Geometry: final body of the model. Coordinates: model frame, mm. Round coordinates to 2 decimals unless told otherwise and drop trailing zeros. Write each loop counter-clockwise with the first axis right and the second up, starting at its lowest first coordinate (ties: lowest second). Pieces come first, ordered by that corner, then holes. Notation, with made-up numbers: (45.25, -1) -> (96.25, -1) arc R12 ccw to (96.25, 12) -> close; hole circle Ø6 at (7.25, 74.25). An arc over 180 degrees is marked (long way). Use one line per item in the form item = value. Start each with the question number.
1. Cut plane B-B, the plane x = 1137.5. Return the cut outline in (y, z) (3 decimals), plus the area to 3 significant figures.
2. Pin query (flat end, axial travel): pin 1 Ø0.6 at (x, z) = (1142.5, 568) entering from +Y; pin 2 Ø3 at (x, y) = (1138, 34) entering from -Z; pin 3 Ø10 at (x, z) = (1132.5, 235.5) entering from -Y. Return the tip coordinate at first contact, or that it passes through.
3. Line query: L1, parallel to X at y = 27, z = 385.5; L2, parallel to Y at x = 1136.75, z = -371 (3 decimals); L3, parallel to Y at x = 1125.5, z = -221.5. Output: solid intervals per line, ascending.
```python
from build123d import *

# Parameters (mm, degrees)
EXTRUDE1_DEPTH     = 599.28125
CUT_EXTRUDE1_DEPTH = 25.4
CUT_EXTRUDE2_DEPTH = 25.4
CUT_EXTRUDE3_DEPTH = 25.4
SKETCH5_W          = 4.7625
SKETCH5_H          = 4.7625
CUT_EXTRUDE4_DEPTH = 0.79375
FILLET1_R          = 6.35


with BuildPart() as part:
    # Sketch1 → Extrude1 (new body, symmetric)
    with BuildSketch(Plane.XY):
        with BuildLine():
            Line((1143, 0), (1142.20625, 0))
            Line((1142.20625, 0), (1142.20625, 32.54375))
            ThreePointArc((1142.20625, 32.54375), (1141.741282015, 33.666282015), (1140.61875, 34.13125))
            Line((1140.61875, 34.13125), (1128.140506397, 34.13125))
            Line((1128.140506397, 34.13125), (1123.091401986, 31.071186722))
            Line((1123.091401986, 31.071186722), (1122.68, 31.75))
            Line((1122.68, 31.75), (1127.91875, 34.925))
            Line((1127.91875, 34.925), (1140.61875, 34.925))
            ThreePointArc((1140.61875, 34.925), (1142.302548023, 34.227548023), (1143, 32.54375))
            Line((1143, 32.54375), (1143, 0))
        make_face()
    extrude(amount=EXTRUDE1_DEPTH, both=True)

    # Sketch2 → Cut-Extrude1 (cut)
    with BuildSketch(Plane(origin=(1143, 0, 0), x_dir=(0, 0, -1), z_dir=(1, 0, 0))):
        Polygon((599.28125, 34.925), (542.13125, 34.925), (542.13125, 31.75), (599.28125, 20.6502), align=None)
        Polygon((-599.28125, 34.925), (-542.13125, 34.925), (-542.13125, 31.75), (-599.28125, 20.6502), align=None)
    extrude(amount=-CUT_EXTRUDE1_DEPTH, mode=Mode.SUBTRACT)

    # Sketch3 → Cut-Extrude2 (cut)
    with BuildSketch(Plane(origin=(0, 0, -542.13125), x_dir=(-1, 0, 0), z_dir=(0, 0, -1))):
        Polygon((-1127.91875, 34.925), (-1122.68, 31.75), (-1123.420434334, 30.528283348), (-1128.140506397, 34.13125), align=None)
    extrude(amount=CUT_EXTRUDE2_DEPTH, mode=Mode.SUBTRACT)

    # Sketch4 → Cut-Extrude3 (cut)
    with BuildSketch(Plane.XY.offset(542.13125)):
        Polygon((1127.91875, 34.925), (1122.68, 31.75), (1124.000635951, 29.570950682), (1128.140506397, 34.13125), align=None)
    extrude(amount=CUT_EXTRUDE3_DEPTH, mode=Mode.SUBTRACT)

    # Sketch5 → Cut-Extrude4 (cut)
    with BuildSketch(Plane(origin=(1143, 0, 0), x_dir=(0, 0, -1), z_dir=(1, 0, 0))):
        with Locations((568.325, 6.62305)):
            Rectangle(SKETCH5_W, SKETCH5_H)
        with Locations((-568.325, 6.62305)):
            Rectangle(SKETCH5_W, SKETCH5_H)
    extrude(amount=-CUT_EXTRUDE4_DEPTH, mode=Mode.SUBTRACT)

    # Fillet1
    fillet1_edges = [part.edges().sort_by_distance(p)[0] for p in [
        (1142.603125, 20.6502, -599.28125),
        (1142.603125, 0, 599.28125),
        (1142.603125, 20.6502, 599.28125),
        (1142.603125, 0, -599.28125),
    ]]
    fillet(fillet1_edges, radius=FILLET1_R)


solid = part.part
```
Outcome:
q1.outline = (34.131, -542.131) -> (34.925, -542.131) -> (34.925, 542.131) -> (34.131, 542.131) -> close
q1.area = 861 mm^2
q2.pin_1 = 26.78
q2.pin_2 = -542.13
q2.pin_3 = 33.74
q3.L1 = 1142.21 to 1143
q3.L2 = 34.131 to 34.925
q3.L3 = 32.53 to 33.46
